Design review of the part built by this model. Coordinates are the model's own, in mm. Face numbers are marked on the shaded views. A direction names the side the tool comes from. Give positions to 0.01 mm unless a question says otherwise; leave off trailing zeros. Order: outer loops, then holes, each group sorted by start corner. A loop starts at its lowest first (then second) coordinate and runs counter-clockwise, first axis right, second up. Notation, with made-up numbers: (73, -2) -> (81, -2) arc R18 ccw to (81, 5) -> close; hole circle Ø7 at (34, -21). An arc over 180 degrees is marked (long way). Return JSON: item names as keys, results as strings.
```python
from build123d import *

# Parameters (mm, degrees)
SKETCH1_W   = 7.08
SKETCH1_H   = 3.133597909
SKETCH1_W_2 = 11.27
SKETCH1_W_3 = 7.05


with BuildPart() as part:
    # Sketch1 → Revolve1 (revolve)
    with BuildSketch(Plane.XY, mode=Mode.PRIVATE) as revolve1_sk:
        with Locations((-8.41, 1.566798955)):
            Rectangle(SKETCH1_W, SKETCH1_H)
        with Locations((0.765, 1.566798955)):
            Rectangle(SKETCH1_W_2, SKETCH1_H)
        Polygon((6.4, 7.11), (0, 7.11), (0, 5.55), (-4.87, 5.55), (-4.87, 3.133597909), (6.4, 3.133597909), align=None)
        with Locations((9.925, 1.566798955)):
            Rectangle(SKETCH1_W_3, SKETCH1_H)
    revolve(revolve1_sk.sketch.rotate(Axis((-4.87, 0, 0), (1, 0, 0)), 180), axis=Axis((-4.87, 0, 0), (1, 0, 0)))


solid = part.part
```
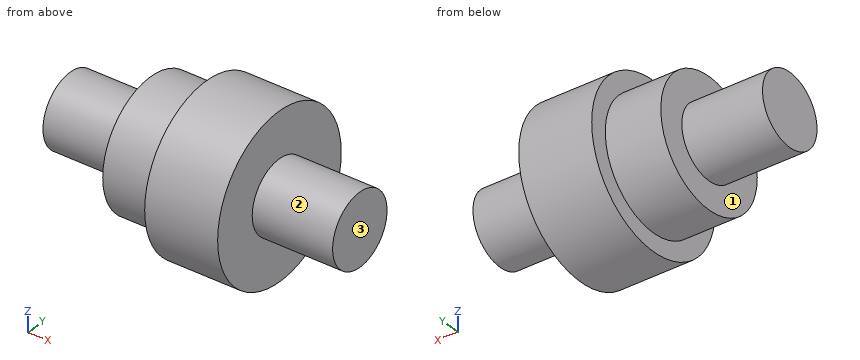
Item 1: Machinability: for the marked faces 1, 2 and 3, which of the approach directions +Z, -Z, +X, -X, +Y, -Y give a long, thin tool a straight path to every point of the face, cutting with its end or side? Answer none if there is none.
Result set:
{"face 1": "-X", "face 2": "+X", "face 3": "+Z, -Z, +X, +Y, -Y"}
Item 2: Add section C-C (x = 7.5). Give the boundary of the cut face in (y, z), plus the area to 3 significant figures.
Result set:
{"outline": "circle Ø6.27 at (0, 0)", "area": "30.8 mm^2"}
Item 3: Add section D-D (z = 4.5). Give the boundary of the cut face in (x, y).
Result set:
{"outline": "(-4.87, -3.25) -> (0, -3.25) -> (0, -5.5) -> (6.4, -5.5) -> (6.4, 5.5) -> (0, 5.5) -> (0, 3.25) -> (-4.87, 3.25) -> close"}
Item 4: Wall thickness on L1, parallel to X at y = -4.5, z = -0.5; L2, parallel to X at y = 5.75, z = 1.25; L3, parallel to Z at x = -9.5, y = 2.25: over which ranges is each line inside the solid? List them lowest first. Write a range as [from, to].
Result set:
{"L1": "x = [-4.87, 6.4]", "L2": "x = [0, 6.4]", "L3": "z = [-2.18, 2.18]"}
Item 5: For pin 1 (6 mm diameter, centred on x = 4, z = -4, fed in from +Y); pin 2 (6 mm diameter, centred on y = -2, z = 3, fed in from +X); pin 3 (3 mm diameter, centred on y = -1.5, z = 5.5, fed in from +X); pin 4 (3 mm diameter, centred on x = 6.5, z = -5.5, fed in from +Y), all flat-tipped, find the tip position at first contact; note any pin that passes through.
Result set:
{"pin 1": "stops at y = 7.04", "pin 2": "stops at x = 13.45", "pin 3": "stops at x = 6.4", "pin 4": "stops at y = 5.88"}
Item 6: Add section A-A (z = 0). Give the boundary of the cut face in (x, y).
Result set:
{"outline": "(-11.95, -3.13) -> (-4.87, -3.13) -> (-4.87, -5.55) -> (0, -5.55) -> (0, -7.11) -> (6.4, -7.11) -> (6.4, -3.13) -> (13.45, -3.13) -> (13.45, 3.13) -> (6.4, 3.13) -> (6.4, 7.11) -> (0, 7.11) -> (0, 5.55) -> (-4.87, 5.55) -> (-4.87, 3.13) -> (-11.95, 3.13) -> close"}
